Solid Edge part; units mm, degrees
sketch "Sketch1" plane through (0, 0, 0) normal (0, 0, 1) x (1, 0, 0)
  line L0 (141.4412, 25.0317) -> (3.3528, 25.0317)
  line L1 (3.3528, 25.0317) -> (3.3528, 1.7653)
  line L2 (3.3528, 1.7653) -> (141.4412, 1.7653)
  line L3 (141.4412, 1.7653) -> (141.4412, 25.0317)
extrude "Protrusion1" add sketch "Sketch1" against normal blind 1.5875
sketch "Sketch2" plane through (72.397, 13.3985, 0) normal (0, 0, 1) x (-1, 0, 0)
  line L0 (-69.0442, 11.6332) -> (-69.0442, -11.6332)
  line L1 (69.0442, -11.6332) -> (-69.0442, -11.6332)
  line L2 (69.0442, -11.6332) -> (69.0442, 11.6332)
  line L3 (67.4694, 11.6332) -> (69.0442, 11.6332)
  line L4 (67.4694, -10.0584) -> (67.4694, 11.6332)
  line L5 (-67.4694, -10.0584) -> (67.4694, -10.0584)
  line L6 (-67.4694, 11.6332) -> (-67.4694, -10.0584)
  line L7 (-69.0442, 11.6332) -> (-67.4694, 11.6332)
extrude "ExtrudedProtrusion_2" add sketch "Sketch2" against normal blind 10.16
For this review, take the finished solid that the model builds, in its own axes (mm). A direction names the side the tool comes from. Round coordinates to 2 decimals unless told otherwise and drop trailing zeros. Write each loop counter-clockwise with the first axis right and the second up, starting at its lowest first coordinate (ties: lowest second). Pieces come first, ordered by that corner, then holes. Notation, with made-up numbers: (79.25, -26) - (137.25, -26) arc R12 ccw to (137.25, -11) - close; hole circle Ø5 at (22.5, 27). An arc over 180 degrees is marked (long way). Put each result on its own line as item: value.
Q1. Insertion check: pin 1 Ø12 at (x, y) = (119.5, 10) entering from -Z; pin 2 Ø4.5 at (x, z) = (99.5, -6.5) entering from -Y. Each pin has a flat end and moves straight along its axis. Give the tip position at first contact, or say it passes through.
Solved:
pin 1: stops at z = -1.59
pin 2: stops at y = 23.46
Q2. Machinability: for faces 5 (the face through (73, 23.457, -6)), 6 (the face through (72, 24, -10.16)), which of the approach directions +Z, -Z, +X, -X, +Y, -Y give a long, thin tool a straight path to every point of the face, cutting with its end or side? Answer none if there is none.
Solved:
face 5: -Z, -Y
face 6: -Z, +X, -X, +Y, -Y
Q3. We need section B-B (y = 15.75). Give the boundary of the cut face in (x, z), and give its area (3 significant figures).
Solved:
outline: (3.35, -10.16) - (4.93, -10.16) - (4.93, -1.59) - (139.87, -1.59) - (139.87, -10.16) - (141.44, -10.16) - (141.44, 0) - (3.35, 0) - close
area: 246 mm2
Q4. We need section C-C (x = 81.5). Give the boundary of the cut face in (y, z), and give its area (3 significant figures).
Solved:
outline: (1.77, -1.59) - (23.46, -1.59) - (23.46, -10.16) - (25.03, -10.16) - (25.03, 0) - (1.77, 0) - close
area: 50.4 mm2
Q5. Wall thickness on probe 1 along X at (y, z) = (22.25, -3.75); probe 2 along Y at (x, z) = (28.5, -7); probe 3 along Z at (x, y) = (39, 22.5): over which ranges is each line inside the solid? List them lowest first.
Solved:
probe 1: x = 3.35 to 4.93, 139.87 to 141.44
probe 2: y = 23.46 to 25.03
probe 3: z = -1.59 to 0
Q6. Mouldability with a two-part tool opening along X and no side actions: class faces 1 (the face through (141.441, 13, -5)), 2 (the face through (139.866, 12, -6)), 3 (the face through (71, 13, -1.588)), 4 (the face through (71, 14, 0)) as released by +X, released by -X, zero draft, split by the parting line, or undercut.
Solved:
face 1: released by +X
face 2: undercut
face 3: undercut
face 4: zero draft
Q7. We need section A-A (z = -6.5). Give the boundary of the cut face in (x, y), and give its area (3 significant figures).
Solved:
outline: (3.35, 1.77) - (4.93, 1.77) - (4.93, 23.46) - (139.87, 23.46) - (139.87, 1.77) - (141.44, 1.77) - (141.44, 25.03) - (3.35, 25.03) - close
area: 286 mm2
